Answer from the drawing. Dimensions are ordinates in mm from the lowest x, y and z of the part. Round coordinates to 2 decimals unless told otherwise and drop trailing zeros. Write each loop counter-clockwise with the first axis right and the second up, starting at its lowest first coordinate (ties: lowest second). Pieces come first, ordered by that corner, then holes. Notation, with made-up numbers: (35.25, 12.25) - (77.25, 12.25) arc R14 ccw to (77.25, 16.25) - close; hole circle Ø7 at (48.25, 45). An arc over 180 degrees is marked (long way). Answer as a JSON object with one key per item and string values.
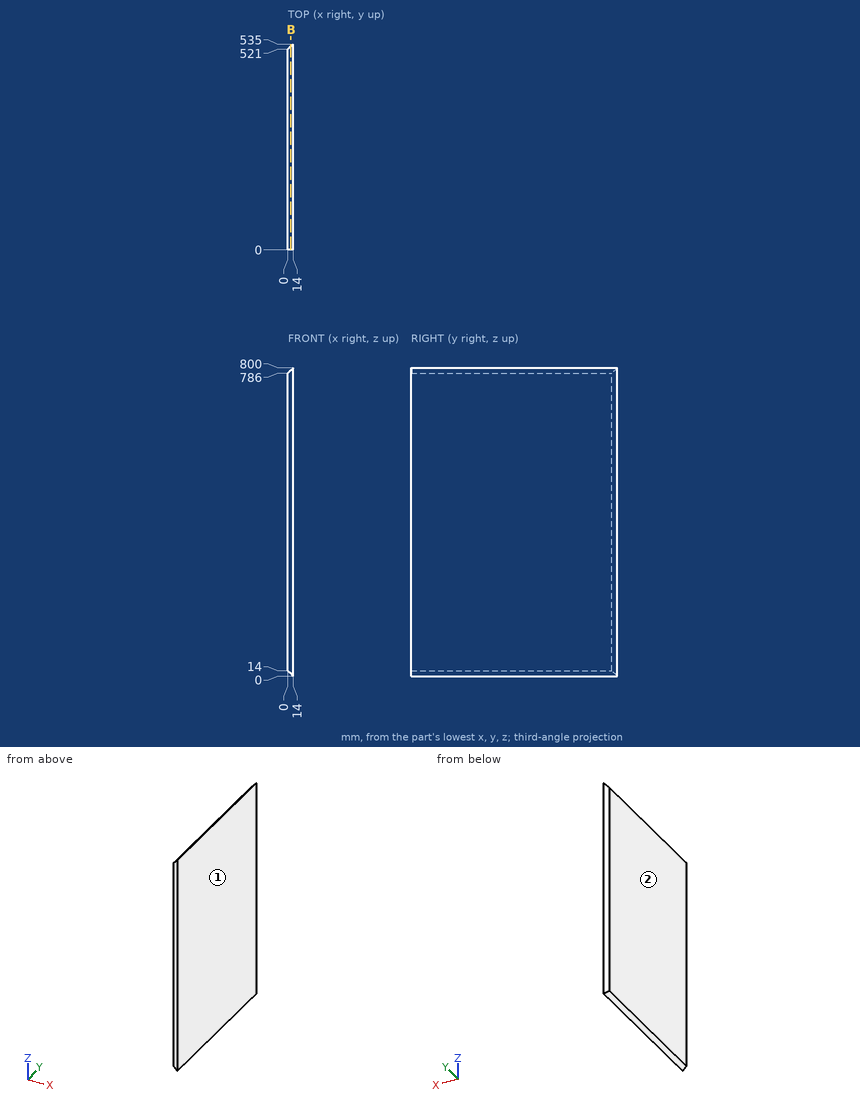
Item 1: A cutting plane is placed at B-B (x = 8.25). Write down the section's boundary in (y, z).
Results found:
{"outline": "(0, 5.75) - (529.25, 5.75) - (529.25, 794.25) - (0, 794.25) - close"}
Item 2: Each of these flat-tipped pins is pushed along its axis until it touches: P1, Ø1.5, axis at x = 2.5, y = 100, coming from the -Z side; P2, Ø8, axis at x = 8.5, y = 434, coming from the -Z side; P3, Ø8, axis at x = 3, y = 438, coming from the +Z side. Where does it stop, or does it pass through?
Results found:
{"P1": "z = 10.75", "P2": "z = 1.5", "P3": "z = 793"}
Item 3: Consider line 1 along Z through (x, y) = (2, 95.5); line 2 along Y through (x, z) = (8, 247.5); line 3 along Z through (x, y) = (5, 160). Determine where each line is inside the solid, lowest interval first.
Results found:
{"line 1": "12 to 788", "line 2": "0 to 529", "line 3": "9 to 791"}
Item 4: Determine the mould class of the marked faces 1 and 2 for opening direction X: pulls with the +X half, pulls with the -X half, needs draft (parallel to the pull), parting line crosses it, or undercut.
Results found:
{"face 1": "pulls with the +X half", "face 2": "pulls with the -X half"}
